Model file for the job. Use its own axes, mm. A direction names the side the tool comes from. Round coordinates to 2 decimals unless told otherwise and drop trailing zeros. Order: outer loops, then holes, each group sorted by start corner. A loop starts at its lowest first (then second) coordinate and runs counter-clockwise, first axis right, second up. Notation, with made-up numbers: (26, 30) - (53, 30) arc R18 cw to (53, 45) - close; hole circle Ø3 at (-39.5, 64.25). An arc over 180 degrees is marked (long way). Put each result on its own line as item: value. Start each with the question number.
Item 1: Pin check, flat tip, straight feed: pin 1 Ø1 at (x, y) = (259, 363.5) entering from +Z. Stop position of the tip, or through.
Item 2: Saw through at C-C on x = 148.5. List the corners of the cut face in (y, z), plus the area to 4 significant figures.
Item 3: Saw through at B-B on y = 181.5. List the corners of the cut face in (x, z).
Item 4: Saw through at A-A on x = -342.5. List the corners of the cut face in (y, z), plus the area to 4 significant figures.
Item 5: Probe probe 1 along Y at (x, z) = (245.5, 470); probe 2 along Z at (x, y) = (-429, -679); probe 3 along X at (y, z) = (479, 480.5). List the from-to ranges inside material, lowest first.
Item 6: Which spindle directions (+Z, -Z, +X, -X, +Y, -Y) get a long thin tool onto all of the face, cutting with end or side? Do faces 1 (the face through (-7, -800, 197)), 2 (the face through (-250, 180, 501)), 3 (the face through (-377, 180, 600)). Say none if no direction does.
Item 7: Saw through at D-D on y = -695.5. List the corners of the cut face in (x, z), plus the area to 3 significant figures.
```python
from build123d import *

# Parameters (mm, degrees)
F0_W     = 1000
F0_H     = 1600
F1_DEPTH = 750
F3_DEPTH = 350
F4_W     = 250
F4_H     = 750
F5_DEPTH = 150


with BuildPart() as f1:
    # F0 (on Top) → F1 (new body)
    with BuildSketch(Plane.XY):
        Rectangle(F0_W, F0_H)
    extrude(amount=F1_DEPTH)

    # F2 (on face) → F3 (cut)
    with BuildSketch(Plane.XY.offset(750)):
        Polygon((-250, -200), (-500, -200), (-500, -800), (500, -800), (500, 550), (-250, 550), align=None)
    extrude(amount=-F3_DEPTH, mode=Mode.SUBTRACT)

    # F4 (on face) → F5 (cut)
    with BuildSketch(Plane.XY.offset(750)):
        with Locations((-375, 175)):
            Rectangle(F4_W, F4_H)
    extrude(amount=-F5_DEPTH, mode=Mode.SUBTRACT)


solid = f1.part
```
Results found:
1. pin 1: stops at z = 400
2. outline: (-800, 0) - (800, 0) - (800, 750) - (550, 750) - (550, 400) - (-800, 400) - close
2. area: 727,500 mm²
3. outline: (-500, 0) - (500, 0) - (500, 400) - (-250, 400) - (-250, 600) - (-500, 600) - close
4. outline: (-800, 0) - (800, 0) - (800, 750) - (550, 750) - (550, 600) - (-200, 600) - (-200, 400) - (-800, 400) - close
4. area: 877,500 mm²
5. probe 1: y = 550 to 800
5. probe 2: z = 0 to 400
5. probe 3: x = -500 to -250
6. face 1: +Z, -Z, +X, -X, -Y
6. face 2: +Z, +X, -Y
6. face 3: +Z, +X, -X, -Y
7. outline: (-500, 0) - (500, 0) - (500, 400) - (-500, 400) - close
7. area: 400,000 mm²
